Build history of the part. All positions in model axes, mm. A direction names the side the tool comes from. Give positions to 0.01 mm unless a question says otherwise; leave off trailing zeros. Order: outer loops, then holes, each group sorted by start corner. A loop starts at its lowest first (then second) coordinate and runs counter-clockwise, first axis right, second up. Notation, with made-up numbers: (12, 28.5) -> (54, 28.5) arc R19 cw to (54, 51.5) -> close; hole circle Ø6 at (41.5, 8). An arc over 180 degrees is marked (long way). One line per item, written item: value. Start each with the question number.
(1) Saw through at C-C on z = 54. Give the cut face in (x, y).
(2) Which spindle directions (+Z, -Z, +X, -X, +Y, -Y) get a long thin tool onto all of the face, cutting with end or side? Do faces 5 (the flat face through (20, 0, 28)), 6 (the flat face through (7, -20, 6)), 7 (the flat face through (0, -8, 65)). Say none if no direction does.
(3) Two-plate mould, pull along X, no slides. Class faces 1 (the flat face through (0, -16, 40)), 2 (the flat face through (-20, 0, 28)), 3 (the flat face through (30, -25, 20)), 4 (the cylindrical face through (-7.493, 0.33, 74.86)): +X half, -X half, draft (parallel to the pull), parting line (faces both ways), or undercut.
(4) Saw through at D-D on x = -10. Give the cut face in (y, z), plus the area to 4 significant figures.
(5) Saw through at B-B on y = 0. Give the cut face in (x, z), plus the area to 4 significant figures.
(6) Probe line 1 (X direction, y = -19, z = 11); line 2 (Y direction, x = 16, z = 6); line 3 (Z direction, x = -12.5, y = -20.5). List the from-to ranges inside material, lowest first.
(7) Pin check, flat tips, straight feed: pin 1 (5 mm diameter, centred on y = -11.5, z = 46, fed in from +X); pin 2 (3 mm diameter, centred on x = -10, y = -1, fed in from +Z); pin 3 (1.5 mm diameter, centred on x = -17, y = -18.5, fed in from -Z). Stop position of each tip, or through.
(8) Saw through at A-A on x = 0. Give the cut face in (y, z), plus the area to 4 significant figures.
```python
from build123d import *

# Parameters (mm, degrees)
EXTRUDE_1_DEPTH     = 40
CUT_EXTRUDE_1_DEPTH = 40
SKETCH_3_R          = 12.5
EXTRUDE_2_DEPTH     = 25
SKETCH_4_R          = 7.5
EXTRUDE_3_DEPTH     = 20


with BuildPart() as part:
    # 草图1 → 凸台-拉伸1 (new body)
    with BuildSketch(Plane.XY):
        Polygon((-20, -20), (-30, -20), (-30, -30), (30, -30), (30, -20), (20, -20), (20, 20), (-20, 20), align=None)
    extrude(amount=EXTRUDE_1_DEPTH)

    # 草图2 → 切除-拉伸1 (cut)
    with BuildSketch(Plane(origin=(20, 0, 0), x_dir=(0, 0, -1), z_dir=(1, 0, 0))):
        Polygon((0, -20), (-10, -20), (-25, 20), (0, 20), align=None)
    extrude(amount=-CUT_EXTRUDE_1_DEPTH, mode=Mode.SUBTRACT)

    # 草图3 → 凸台-拉伸2 (add)
    with BuildSketch(Plane.XY.offset(40)):
        Circle(SKETCH_3_R)
    extrude(amount=EXTRUDE_2_DEPTH)

    # 草图4 → 凸台-拉伸3 (add)
    with BuildSketch(Plane.XY.offset(65)):
        Circle(SKETCH_4_R)
    extrude(amount=EXTRUDE_3_DEPTH)


solid = part.part
```
Results below:
1. outline: circle Ø25 at (0, 0)
2. face 5: +Z, -Z, +X, +Y
2. face 6: -Z, +Y
2. face 7: +Z
3. face 1: draft
3. face 2: -X half
3. face 3: +X half
3. face 4: parting line
4. outline: (-30, 0) -> (-20, 0) -> (-20, 10) -> (20, 25) -> (20, 40) -> (7.5, 40) -> (7.5, 65) -> (-7.5, 65) -> (-7.5, 40) -> (-30, 40) -> close
4. area: 1,675 mm²
5. outline: (-20, 17.5) -> (20, 17.5) -> (20, 40) -> (12.5, 40) -> (12.5, 65) -> (7.5, 65) -> (7.5, 85) -> (-7.5, 85) -> (-7.5, 65) -> (-12.5, 65) -> (-12.5, 40) -> (-20, 40) -> close
5. area: 1,825 mm²
6. line 1: x = -20 to 20
6. line 2: y = -30 to -20
6. line 3: z = 0 to 40
7. pin 1: stops at x = 8.67
7. pin 2: stops at z = 65
7. pin 3: stops at z = 10.28
8. outline: (-30, 0) -> (-20, 0) -> (-20, 10) -> (20, 25) -> (20, 40) -> (12.5, 40) -> (12.5, 65) -> (7.5, 65) -> (7.5, 85) -> (-7.5, 85) -> (-7.5, 65) -> (-12.5, 65) -> (-12.5, 40) -> (-30, 40) -> close
8. area: 2,225 mm²
